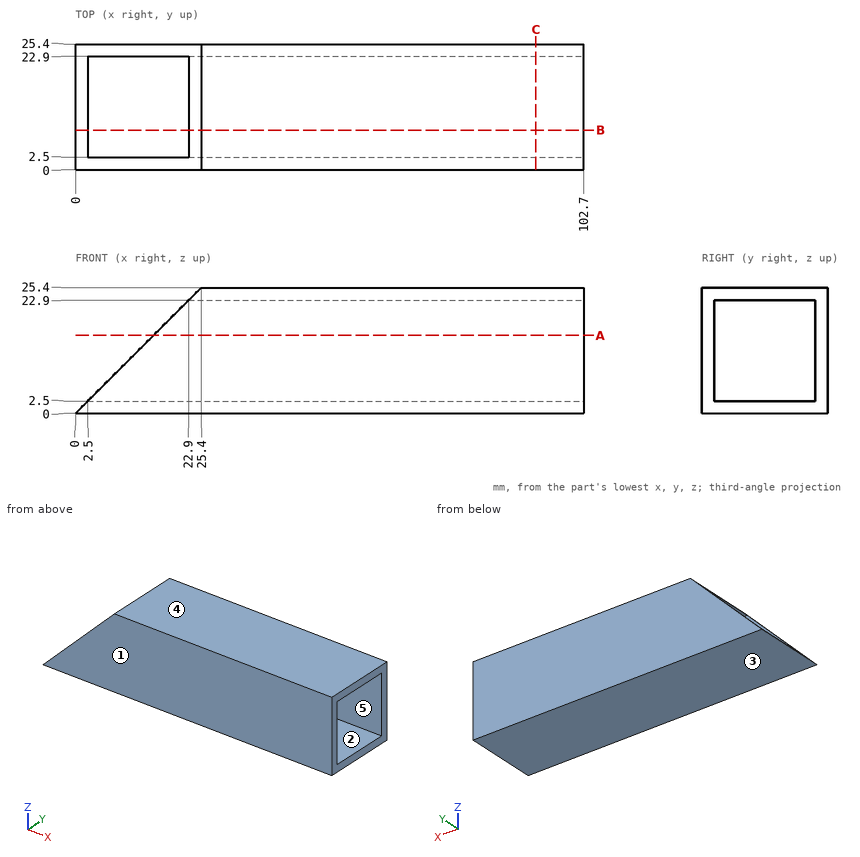
Design review of the part shown in the three views and the two pictorial views. Dimensions are in mm from the part's minimum x, y and z. A direction names the side the tool comes from. Coordinates: 2 decimals unless noted, no trailing zeros. Order: outer loops, then holes, each group sorted by start corner. A loop starts at its lowest first (then second) coordinate and runs counter-clockwise, first axis right, second up.
1) Take a section at C-C, the plane x = 93. Give the boundary of the cut face in (y, z), and give its area (3 significant figures).
2) Take a section at A-A, the plane z = 15.75. Give the boundary of the cut face in (x, y).
3) Mouldability with a two-part tool opening along Y and no side actions: class the marked faces 1, 2 and 3 as +Y half, -Y half, draft (parallel to the pull), parting line (faces both ways), or undercut.
4) Take a section at B-B, the plane y = 8. Give the boundary of the cut face in (x, z).
5) For the marked faces 4 and 5, list the 3-axis set-ups (+Z, -Z, +X, -X, +Y, -Y) from which the entire face can be reached by the end or side of a thin tool; tool diameter is ignored.
6) Wall thickness on line 1 along Z through (x, y) = (66, 6.5); line 2 along Z through (x, y) = (24, 12.75): over which ranges is each line inside the solid? List them lowest first.
Returned:
1. outline: (0, 0) - (25.4, 0) - (25.4, 25.4) - (0, 25.4) - close; hole (2.5, 2.5) - (22.9, 2.5) - (22.9, 22.9) - (2.5, 22.9) - close
1. area: 229 mm2
2. outline: (15.75, 0) - (102.7, 0) - (102.7, 2.5) - (15.75, 2.5) - close; (15.75, 22.9) - (102.7, 22.9) - (102.7, 25.4) - (15.75, 25.4) - close
3. face 1: -Y half
3. face 2: undercut
3. face 3: draft
4. outline: (0, 0) - (102.7, 0) - (102.7, 2.5) - (2.5, 2.5) - close; (22.9, 22.9) - (102.7, 22.9) - (102.7, 25.4) - (25.4, 25.4) - close
5. face 4: +Z, +X, -X, +Y, -Y
5. face 5: +X, -X
6. line 1: z = 0 to 2.5, 22.9 to 25.4
6. line 2: z = 0 to 2.5, 22.9 to 24
